from build123d import *

# Parameters (mm, degrees)
SKETCH1_W             = 117.475
SKETCH1_H             = 19.05
BOSS_EXTRUDE1_DEPTH   = 9.525
BOSS_EXTRUDE2_DEPTH   = 3.175
F_6_CLEARANCE_HOLE1_D = 4.3053
SKETCH5_W             = 12.065
SKETCH5_H             = 12.065
CUT_EXTRUDE1_DEPTH    = 10.525
SKETCH7_W             = 116.205
SKETCH7_H             = 14.605
CUT_EXTRUDE2_DEPTH    = 7.9502
SKETCH8_W             = 117.475
SKETCH8_H             = 28.575
CUT_EXTRUDE3_DEPTH    = 3.175
FILLET2_R             = 1.27
FILLET3_R             = 0.762
FILLET4_R             = 0.508
FILLET5_R             = 0.508


with BuildPart() as part:
    # Sketch1 → Boss-Extrude1 (new body)
    with BuildSketch(Plane.XY):
        with Locations((0, -57.6104797)):
            Rectangle(SKETCH1_W, SKETCH1_H)
    extrude(amount=BOSS_EXTRUDE1_DEPTH)

    # Sketch2 → Boss-Extrude2 (add)
    with BuildSketch(Plane.XY):
        with BuildLine():
            Line((35.56, -48.0854797), (58.7375, -48.0854797))
            Line((58.7375, -48.0854797), (44.939976119, -39.26086832))
            ThreePointArc((44.939976119, -39.26086832), (40.410479427, -39.106525106), (38.1, -43.0054797))
            Line((38.1, -43.0054797), (38.1, -45.5454797))
            ThreePointArc((38.1, -45.5454797), (37.356051224, -47.341530924), (35.56, -48.0854797))
        make_face()
        with BuildLine():
            Line((-38.1, -45.5454797), (-38.1, -43.0054797))
            ThreePointArc((-38.1, -43.0054797), (-40.410479427, -39.106525106), (-44.939976119, -39.26086832))
            Line((-44.939976119, -39.26086832), (-58.7375, -48.0854797))
            Line((-58.7375, -48.0854797), (-35.56, -48.0854797))
            ThreePointArc((-35.56, -48.0854797), (-37.356051224, -47.341530924), (-38.1, -45.5454797))
        make_face()
    extrude(amount=BOSS_EXTRUDE2_DEPTH)

    # #6 Clearance Hole1 (through all)
    with Locations(Plane.XY.offset(3.175)):
        with Locations((42.545, -43.0054797), (-42.545, -43.0054797)):
            Hole(F_6_CLEARANCE_HOLE1_D / 2)

    # Sketch5 → Cut-Extrude1 (cut, through all)
    with BuildSketch(Plane.XY.offset(9.525)):
        with Locations((50.8, -56.6198797)):
            Rectangle(SKETCH5_W, SKETCH5_H)
        with Locations((33.866666667, -56.6198797)):
            Rectangle(SKETCH5_W, SKETCH5_H)
        with Locations((16.933333333, -56.6198797)):
            Rectangle(SKETCH5_W, SKETCH5_H)
        with Locations((0, -56.6198797)):
            Rectangle(SKETCH5_W, SKETCH5_H)
        with Locations((-16.933333333, -56.6198797)):
            Rectangle(SKETCH5_W, SKETCH5_H)
        with Locations((-33.866666667, -56.6198797)):
            Rectangle(SKETCH5_W, SKETCH5_H)
        with Locations((-50.8, -56.6198797)):
            Rectangle(SKETCH5_W, SKETCH5_H)
    extrude(amount=-CUT_EXTRUDE1_DEPTH, mode=Mode.SUBTRACT)

    # Sketch7 → Cut-Extrude2 (cut)
    with BuildSketch(Plane(origin=(0, 0, 0), x_dir=(-1, 0, 0), z_dir=(0, 0, -1))):
        with Locations((0, -56.6198797)):
            Rectangle(SKETCH7_W, SKETCH7_H)
    extrude(amount=-CUT_EXTRUDE2_DEPTH, mode=Mode.SUBTRACT)

    # Sketch8 → Cut-Extrude3 (cut)
    with BuildSketch(Plane(origin=(0, 0, 0), x_dir=(-1, 0, 0), z_dir=(0, 0, -1))):
        with Locations((0, -52.8479797)):
            Rectangle(SKETCH8_W, SKETCH8_H)
    extrude(amount=-CUT_EXTRUDE3_DEPTH, mode=Mode.SUBTRACT)

    # Fillet2
    fillet2_edges = [part.edges().sort_by_distance(p)[0] for p in [
        (58.7375, -67.1354797, 6.35),
        (58.7375, -48.0854797, 6.35),
        (-58.7375, -48.0854797, 6.35),
        (-58.7375, -67.1354797, 6.35),
    ]]
    fillet(fillet2_edges, radius=FILLET2_R)

    # Fillet3
    fillet3_edges = [part.edges().sort_by_distance(p)[0] for p in [
        (-58.7375, -57.6104797, 9.525),
        (0, -48.0854797, 9.525),
        (0, -67.1354797, 9.525),
        (58.7375, -57.6104797, 9.525),
        (58.365525612, -66.763505312, 9.525),
        (58.365525612, -48.457454088, 9.525),
        (-58.365525612, -66.763505312, 9.525),
        (-58.365525612, -48.457454088, 9.525),
    ]]
    fillet(fillet3_edges, radius=FILLET3_R)

    # Fillet4
    fillet4_edges = [part.edges().sort_by_distance(p)[0] for p in [
        (0, -63.9223797, 7.9502),
        (-58.1025, -63.9223797, 5.5626),
        (-58.1025, -56.6198797, 7.9502),
        (-58.1025, -49.3173797, 5.5626),
        (0, -49.3173797, 7.9502),
        (58.1025, -49.3173797, 5.5626),
        (58.1025, -56.6198797, 7.9502),
        (58.1025, -63.9223797, 5.5626),
    ]]
    fillet(fillet4_edges, radius=FILLET4_R)

    # Fillet5
    fillet5_edges = [part.edges().sort_by_distance(p)[0] for p in [
        (-56.8325, -50.5873797, 8.7376),
        (-44.7675, -50.5873797, 8.7376),
        (-56.8325, -62.6523797, 8.7376),
        (-44.7675, -62.6523797, 8.7376),
        (-39.899166667, -50.5873797, 8.7376),
        (-27.834166667, -50.5873797, 8.7376),
        (-39.899166667, -62.6523797, 8.7376),
        (-27.834166667, -62.6523797, 8.7376),
        (-22.965833333, -50.5873797, 8.7376),
        (-10.900833333, -50.5873797, 8.7376),
        (-22.965833333, -62.6523797, 8.7376),
        (-10.900833333, -62.6523797, 8.7376),
        (-6.0325, -50.5873797, 8.7376),
        (6.0325, -50.5873797, 8.7376),
        (-6.0325, -62.6523797, 8.7376),
        (6.0325, -62.6523797, 8.7376),
        (10.900833333, -62.6523797, 8.7376),
        (10.900833333, -50.5873797, 8.7376),
        (22.965833333, -62.6523797, 8.7376),
        (22.965833333, -50.5873797, 8.7376),
        (39.899166667, -50.5873797, 8.7376),
        (39.899166667, -62.6523797, 8.7376),
        (27.834166667, -50.5873797, 8.7376),
        (27.834166667, -62.6523797, 8.7376),
        (44.7675, -50.5873797, 8.7376),
        (56.8325, -50.5873797, 8.7376),
        (44.7675, -62.6523797, 8.7376),
        (56.8325, -62.6523797, 8.7376),
    ]]
    fillet(fillet5_edges, radius=FILLET5_R)


solid = part.part
The listing builds one solid part. Answer for the finished solid, in the listing's coordinates (mm). A direction names the side the tool comes from. Round coordinates to 2 decimals unless told otherwise and drop trailing zeros. Loops run counter-clockwise (first coordinate to the right, second up) from the corner with the lowest first, then second, coordinate; pieces in that order, holes last. Notation, with made-up numbers: M 58,-4 L 75,-4 A36 ccw 75,32 Z; hole C 64,43.5 d9. An arc over 180 degrees is marked long. Return JSON: item names as keys, results as strings.
Q1. The mould has two halves that part along Y. Classify faces 3 (the face through (58.102, -57, 5)), 4 (the face through (-1, -67.135, 6)), 5 (the face through (-1, -48.085, 6)): released by +Y, released by -Y, zero draft, split by the parting line, or undercut.
Results list:
{"face 3": "undercut", "face 4": "released by -Y", "face 5": "released by +Y"}
Q2. Find section A-A, the plane x = 35. Determine the outline of the cut face in (y, z) (3 decimals).
Results list:
{"outline": "M -67.135,3.175 L -63.922,3.175 L -63.922,7.442 A0.508 cw -63.414,7.95 L -62.652,7.95 L -62.652,9.525 L -66.373,9.525 A0.762 ccw -67.135,8.763 Z; M -50.587,7.95 L -49.825,7.95 A0.508 cw -49.317,7.442 L -49.317,3.175 L -48.085,3.175 L -48.085,8.763 A0.762 ccw -48.847,9.525 L -50.587,9.525 Z"}
Q3. Find the intervals of material crossed by line 1 along Y through (x, z) = (17, 4.75); line 2 along X through (y, z) = (-58, 6); line 3 along Z through (x, y) = (-39.5, -50.5) (3 decimals), in increasing order. Write a range as from..to.
Results list:
{"line 1": "y = -67.14..-63.92, -49.32..-48.09", "line 2": "x = -58.74..-58.1, 58.1..58.74", "line 3": "z = 7.95..9.525"}
Q4. Find section B-B, the plane z = 5. Determine the outline of the cut face in (x, y).
Results list:
{"outline": "M -58.74,-65.87 A1.27 ccw -57.47,-67.14 L 57.47,-67.14 A1.27 ccw 58.74,-65.87 L 58.74,-49.36 A1.27 ccw 57.47,-48.09 L -57.47,-48.09 A1.27 ccw -58.74,-49.36 Z; hole M -58.1,-63.41 A0.51 ccw -57.59,-63.92 L 57.59,-63.92 A0.51 ccw 58.1,-63.41 L 58.1,-49.83 A0.51 ccw 57.59,-49.32 L -57.59,-49.32 A0.51 ccw -58.1,-49.83 Z"}
Q5. Find section D-D, the plane y = -58.5. State how many separate pieces and enclosed holes the cut face has, plus the area to 3 significant figures.
Results list:
{"separate pieces": "8", "enclosed holes": "0", "area": "57.9 mm2"}
Q6. Which of the six approach directions +Z, -Z, +X, -X, +Y, -Y give full straight-line access (tool end or side, diameter ignored) to faces 1 (the face through (-1, -63, 9.525)), 2 (the face through (0, -50, 7.95))?
Results list:
{"face 1": "+Z, +X, -X, +Y, -Y", "face 2": "-Z"}
Q7. This flat-tipped pin is pushed along its axis until it touches: pin 1 Ø1.5 at (x, y) = (39.5, -56) entering from -Z. Where does it stop, or does it pass through?
Results list:
{"pin 1": "stops at z = 7.95"}
Q8. Find section C-C, the plane x = 8.5. Determine the outline of the cut face in (y, z) (3 decimals).
Results list:
{"outline": "M -67.135,3.175 L -63.922,3.175 L -63.922,7.442 A0.508 cw -63.414,7.95 L -49.825,7.95 A0.508 cw -49.317,7.442 L -49.317,3.175 L -48.085,3.175 L -48.085,8.763 A0.762 ccw -48.847,9.525 L -66.373,9.525 A0.762 ccw -67.135,8.763 Z"}
